Model file for the job. Use its own axes, mm. A direction names the side the tool comes from. Give positions to 0.01 mm unless a question says otherwise; leave off trailing zeros. Loops run counter-clockwise (first coordinate to the right, second up) from the corner with the lowest first, then second, coordinate; pieces in that order, holes last. Notation, with made-up numbers: (-26.75, -10) - (31.25, -10) arc R21 cw to (31.25, 12) - close; hole circle Ø1 at (40, -15). An arc over 180 degrees is marked (long way). Use a Markdown table: item, result.
from build123d import *

# Parameters (mm, degrees)
F0_R     = 1
F1_DEPTH = 2
F2_W     = 46.8014790542
F2_H     = 17
F2_H_2   = 2
F2_H_3   = 42
F3_DEPTH = 2


with BuildPart() as f1:
    # F0 (on Front) → F1 (new body)
    with BuildSketch(Plane.XZ):
        with BuildLine():
            ThreePointArc((0, -2.5), (-2.5, 0), (0, 2.5))
            Line((0, 2.5), (-25, 2.5))
            Line((-25, 2.5), (-61.1211777337, -27.2596868397))
            Line((-61.1211777337, -27.2596868397), (-56.5739951013, -27.3005926817))
            Line((-56.5739951013, -27.3005926817), (-23.0573490262, -2.5))
            Line((-23.0573490262, -2.5), (0, -2.5))
        make_face()
        with BuildLine():
            ThreePointArc((0, -2.5), (1.767766953, -1.767766953), (2.5, 0))
            ThreePointArc((2.5, 0), (1.767766953, 1.767766953), (0, 2.5))
            ThreePointArc((0, 2.5), (-2.5, 0), (0, -2.5))
        make_face()
        Circle(F0_R, mode=Mode.SUBTRACT)
    extrude(amount=F1_DEPTH)

    # F2 (on face) → F3 (join)
    with BuildSketch(Plane(origin=(-11.3351925365, 0, 13.7582262361), x_dir=(0.7717956454, 0, 0.6358706486), z_dir=(-0.6358706486, 0, 0.7717956454))):
        with Locations((-41.1059540414, 8.5)):
            Rectangle(F2_W, F2_H)
        with Locations((-41.1059540414, -1)):
            Rectangle(F2_W, F2_H_2)
        with Locations((-41.1059540414, -23)):
            Rectangle(F2_W, F2_H_3)
    extrude(amount=F3_DEPTH)


solid = f1.part
(1) Pin check, flat tips, straight feed: P1, Ø4, axis at y = 4, z = -23, coming from the +X side; P2, Ø2, axis at y = -1.5, z = -12, coming from the +X side; P3, Ø6, axis at y = -6, z = -6.5, coming from the -X side. Stop position of each tip, or through.
Computed:
| item | result |
|---|---|
| P1 | x = -53.52 |
| P2 | x = -34.54 |
| P3 | x = -42.71 |
(2) Slice it at A-A, the plane y = -26. Write the cut outline in (x, z), plus the area to 3 significant figures.
Computed:
| item | result |
|---|---|
| outline | (-62.39, -25.72) - (-61.12, -27.26) - (-25, 2.5) - (-26.27, 4.04) - close |
| area | 93.6 mm² |
(3) Drill centre lines: probe 1 along Z at (x, y) = (0, -1); probe 2 along Y at (x, z) = (-21.5, -1); probe 3 along X at (y, z) = (-9, 1.5). Where is each one in solid material? Low to high. Write a range as [from, to].
Computed:
| item | result |
|---|---|
| probe 1 | [-2.5, -1], [1, 2.5] |
| probe 2 | [-2, 0] |
| probe 3 | [-29.36, -26.21] |
(4) Slice it at D-D, the plane x = -21. Write the cut outline in (y, z), plus the area to 3 significant figures.
Computed:
| item | result |
|---|---|
| outline | (-2, -2.5) - (0, -2.5) - (0, 2.5) - (-2, 2.5) - close |
| area | 10.0 mm² |
(5) 3-axis set-ups, long thin cutter, end or side, ignore diameter. For faces 1 (the cylindrical face through (0, -1, -1)), 2 (the flat face through (-43.313, -22.706, -12.588)), 3 (the flat face through (-12, -1, -2.5)), 4 (the flat face through (-12, -1, 2.5)), 5 (the flat face through (-29.5, 0, -6.8)): which of +Z, -Z, +X, -X, +Y, -Y reach the whole face in a straight line?
Computed:
| item | result |
|---|---|
| face 1 | +Y, -Y |
| face 2 | -Z, +X, -Y |
| face 3 | -Z, +X, +Y, -Y |
| face 4 | +Z, +X, +Y, -Y |
| face 5 | -Z, +X, +Y |
(6) Slice it at B-B, the plane x = -30.5. Write the cut outline in (y, z).
Computed:
| item | result |
|---|---|
| outline | (-44, -2.03) - (-2, -2.03) - (-2, -8.01) - (0, -8.01) - (0, -2.03) - (17, -2.03) - (17, 0.56) - (-44, 0.56) - close |
(7) Slice it at C-C, the plane z = -4. Write the cut outline in (x, y), plus the area to 3 significant figures.
Computed:
| item | result |
|---|---|
| outline | (-36.03, -44) - (-32.89, -44) - (-32.89, -2) - (-25.08, -2) - (-25.08, 0) - (-32.89, 0) - (-32.89, 17) - (-36.03, 17) - close |
| area | 207 mm² |
